Input: dimensioned drawing with shaded views. Units: mm. Origin: part minimum x, y, z. A direction names the side the tool comes from. Round coordinates to 2 decimals unless told otherwise and drop trailing zeros. Loops run counter-clockwise (first coordinate to the right, second up) from the corner with the lowest first, then second, coordinate; pieces in that order, holes last. Notation, with made-up numbers: M -1,-1 L 24,-1 A7 ccw 24,4 Z; hole C -10,25.25 d5. An arc over 180 degrees is marked long. Put each result on its own line as item: value. Start each with the question number.
1) Section A-A on y = 17.65. Output: boundary loops of the cut face in (x, z), plus the area to 3 significant figures.
2) Pin query (flat end, axial travel): pin 1 (5 mm diameter, centred on y = 28, z = 14, fed in from +X); pin 2 (2 mm diameter, centred on y = 18.5, z = 5.5, fed in from -X); pin 3 (8 mm diameter, centred on x = 23.5, y = 12, fed in from +Z). Return the tip coordinate at first contact, or that it passes through.
3) Section B-B on x = 11. Output: boundary loops of the cut face in (y, z).
4) Reachability of the marked faces 1, 2 and 3 from +Z, -Z, +X, -X, +Y, -Y: full face, straight path, thin tool, end or side. Return the list, or none.
5) Section D-D on x = 4.5. Output: boundary loops of the cut face in (y, z), plus the area to 3 significant figures.
6) Line query: probe 1 along X at (y, z) = (8, 7.5); probe 2 along Z at (x, y) = (11, 17); probe 3 along X at (y, z) = (14, 20). Output: solid intervals per line, ascending.
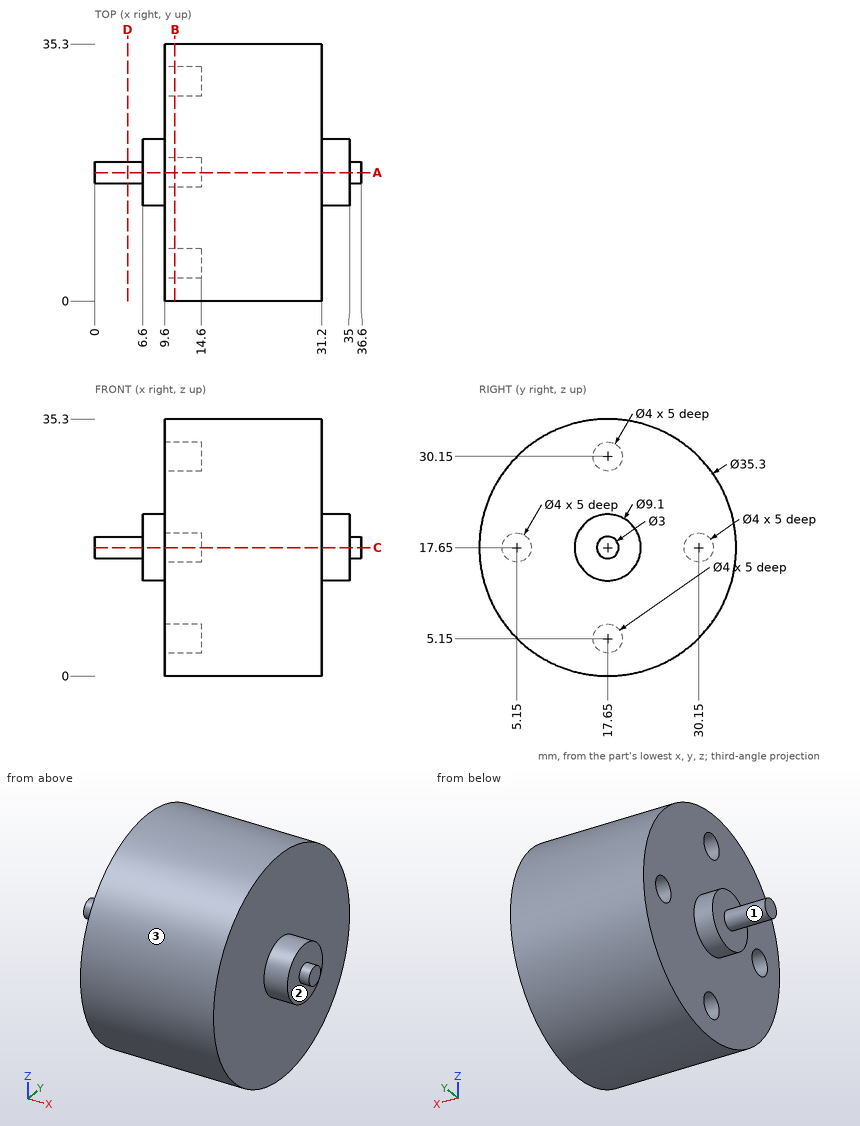
Geometry results:
1. outline: M 0,16.15 L 6.6,16.15 L 6.6,13.1 L 9.6,13.1 L 9.6,7.15 L 14.6,7.15 L 14.6,3.15 L 9.6,3.15 L 9.6,0 L 31.2,0 L 31.2,13.1 L 35,13.1 L 35,16.15 L 36.6,16.15 L 36.6,19.15 L 35,19.15 L 35,22.2 L 31.2,22.2 L 31.2,35.3 L 9.6,35.3 L 9.6,32.15 L 14.6,32.15 L 14.6,28.15 L 9.6,28.15 L 9.6,22.2 L 6.6,22.2 L 6.6,19.15 L 0,19.15 Z
1. area: 809 mm²
2. pin 1: stops at x = 31.2
2. pin 2: stops at x = 14.6
2. pin 3: stops at z = 35.22
3. outline: C 17.65,17.65 d35.3; hole C 5.15,17.65 d4; hole C 17.65,5.15 d4; hole C 17.65,30.15 d4; hole C 30.15,17.65 d4
4. face 1: -X
4. face 2: +X
4. face 3: +X, -X
5. outline: C 17.65,17.65 d3
5. area: 7.07 mm²
6. probe 1: x = 9.6 to 31.2
6. probe 2: z = 0.01 to 3.26, 7.04 to 28.26, 32.04 to 35.29
6. probe 3: x = 6.6 to 35
